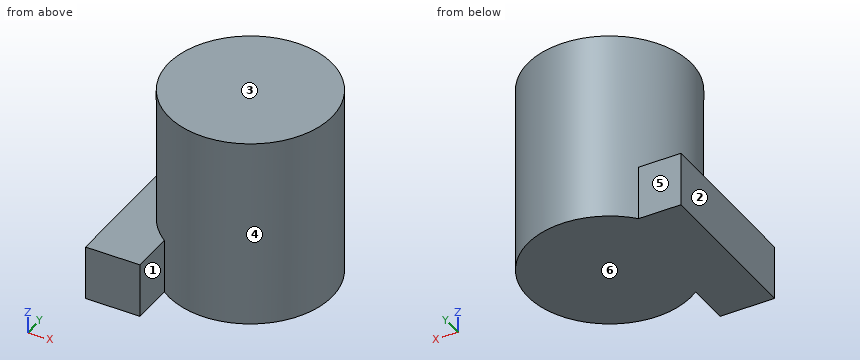
from build123d import *

# Parameters (mm, degrees)
F0_R     = 30
F1_DEPTH = 70
F2_W     = 20
F2_H     = 20
F3_DEPTH = 60


with BuildPart() as f1:
    # F0 (on Top) → F1 (new body)
    with BuildSketch(Plane.XY):
        with Locations((17.760798, -20.20311)):
            Circle(F0_R)
    extrude(amount=F1_DEPTH)

    # F2 (on Front) → F3 (join)
    with BuildSketch(Plane.XZ):
        with Locations((-10, 10)):
            Rectangle(F2_W, F2_H)
    extrude(amount=F3_DEPTH)


solid = f1.part
Geometry: final body of the model. Coordinates: model frame, mm. Face numbers are marked on the shaded views. A direction names the side the tool comes from. Give positions to 0.01 mm unless a question says otherwise; leave off trailing zeros. Order: outer loops, then holes, each group sorted by start corner. A loop starts at its lowest first (then second) coordinate and runs counter-clockwise, first axis right, second up. Notation, with made-up numbers: (50, 33) -> (62, 33) arc R13 cw to (62, 39) -> close; hole circle Ø2 at (11.5, 56). An arc over 180 degrees is marked (long way). Write each question's results on one line, items separated by ' | '.
1) Draft query along X for the marked faces 1, 2 and 3. Return one class per face: released by +X, released by -X, zero draft, split by the parting line, or undercut.
Geometry says:
face 1: undercut | face 2: released by -X | face 3: zero draft
2) Cut plane A-A (z = 13). Output: boundary loops of the cut face in (x, y), and give its area (3 significant figures).
Geometry says:
outline: (-20, -60) -> (0, -60) -> (0, -44.38) arc R30 ccw (long way) to (-4.42, 0) -> (-20, 0) -> close | area: 3,620 mm²
3) Line query: line 1 along Z through (x, y) = (-14.5, -11.5); line 2 along Y through (x, z) = (-14, 7); line 3 along X through (y, z) = (-4.5, 58.5). Output: solid intervals per line, ascending.
Geometry says:
line 1: z = 0 to 20 | line 2: y = -60 to 0 | line 3: x = -7.8 to 43.32
4) Cut plane B-B (x = -7.5). Output: boundary loops of the cut face in (y, z).
Geometry says:
outline: (-60, 0) -> (0, 0) -> (0, 20) -> (-4.02, 20) -> (-4.02, 70) -> (-36.39, 70) -> (-36.39, 20) -> (-60, 20) -> close
5) Cut plane C-C (y = -24). Output: boundary loops of the cut face in (x, z).
Geometry says:
outline: (-20, 0) -> (47.52, 0) -> (47.52, 70) -> (-12, 70) -> (-12, 20) -> (-20, 20) -> close
6) First-contact query: pin 1 Ø1.5 at (y, z) = (0, 29) entering from -X; pin 2 Ø6 at (x, z) = (12.5, 44) entering from -Y; pin 3 Ø2 at (y, z) = (-9, 25) entering from -X. Flat tips, straight axial feed; report the tip coordinate or a pass-through.
Geometry says:
pin 1: stops at x = -5.08 | pin 2: stops at y = -50.12 | pin 3: stops at x = -10.45
7) Cut plane D-D (x = -14.5). Output: boundary loops of the cut face in (y, z).
Geometry says:
outline: (-60, 0) -> (0, 0) -> (0, 20) -> (-60, 20) -> close
8) Set-up query: the marked faces 4, 5 and 6. Return all of +Z, -Z, +X, -X, +Y, -Y with unobstructed straight access to the full face (end or side cutting, diameter ignored); none if empty.
Geometry says:
face 4: +Z | face 5: +Z, -Z, -X, +Y | face 6: -Z, +X, -X, +Y, -Y
